```python
from build123d import *

# Parameters (mm, degrees)
F0_W          = 101.6
F0_H          = 76.2
F2_DEPTH      = 3.81
F3_DEPTH      = 38.1
F3_DEPTH_BACK = 38.1
F5_DEPTH      = 101.6
F6_R          = 2.032
F7_DEPTH      = 25.4
F9_R          = 3.175
F9_R_2        = 2.032
F10_DEPTH     = 25.4
F11_W         = 35.56
F11_H         = 25.4
F12_DEPTH     = 25.4
F13_T1_DEPTH  = 102.3282991577
F13_T3_DEPTH  = 70.6700590666
F13_T5_DEPTH  = 34.6541495789
F13_T11_DEPTH = 70.6700590666
F13_T16_DEPTH = 47.7182991577
F14_SIZE      = 5.08
F15_T1_DEPTH  = 71.0624204228
F15_T3_DEPTH  = 110.5507880402
F15_T5_DEPTH  = 71.0624204227
F16_R         = 5.08


# Not quite as in the source:
# - a fillet or chamfer that OpenCascade refuses, or shapes differently, is made with other operations: its cross-section is extruded or revolved along the edge and cut away or added


with BuildPart() as f2:
    # F0 (on Top) → F2 (new body)
    with BuildSketch(Plane.XY):
        with Locations((-38.1367237687, 0)):
            Rectangle(F0_W, F0_H)
    extrude(amount=F2_DEPTH)

    # F1 (on Front) → F3 (join, two sides)
    with BuildSketch(Plane.XZ) as f3_sk:
        Polygon((-44.9426332565, 25.4), (-88.9367237687, 0), (-44.9426332565, 0), align=None)
    extrude(amount=F3_DEPTH)
    extrude(f3_sk.sketch, amount=-F3_DEPTH_BACK)

    # F4 (on face) → F5 (cut)
    with BuildSketch(Plane.XZ.offset(38.1)):
        Polygon((-88.9367237687, 0), (-82.3376101919, 3.81), (-88.9367237687, 3.81), align=None)
    extrude(amount=-F5_DEPTH, mode=Mode.SUBTRACT)

    # F6 (on face) → F7 (cut)
    with BuildSketch(Plane(origin=(-22.2341809422, 0, 38.5107310565), x_dir=(0.8660254038, 0, 0.5), z_dir=(-0.5, 0, 0.8660254038))):
        with Locations((-69.4014621131, -13.4874)):
            Circle(F6_R)
        with Locations((-69.4014621131, -5.588)):
            Circle(F6_R)
        with Locations((-69.4014621131, 5.5626)):
            Circle(F6_R)
        with Locations((-69.4014621131, 13.462)):
            Circle(F6_R)
        with Locations((-42.4520621131, 13.462)):
            Circle(F6_R)
        with Locations((-42.4520621131, -5.588)):
            Circle(F6_R)
        with Locations((-42.4520621131, -13.4874)):
            Circle(F6_R)
        with Locations((-42.4520621131, 5.5626)):
            Circle(F6_R)
    extrude(amount=-F7_DEPTH, mode=Mode.SUBTRACT)

    # F9 (on offset) → F10 (cut)
    with BuildSketch(Plane(origin=(-20.3291809422, 0, 35.2111742681), x_dir=(0.8660254038, 0, 0.5), z_dir=(-0.5, 0, 0.8660254038))):
        with Locations((-69.4014621131, 13.462)):
            Circle(F9_R)
        with Locations((-69.4014621131, 13.462)):
            Circle(F9_R_2, mode=Mode.SUBTRACT)
        with Locations((-69.4014621131, 5.5626)):
            Circle(F9_R)
        with Locations((-69.4014621131, 5.5626)):
            Circle(F9_R_2, mode=Mode.SUBTRACT)
        with Locations((-69.4014621131, -5.588)):
            Circle(F9_R)
        with Locations((-69.4014621131, -5.588)):
            Circle(F9_R_2, mode=Mode.SUBTRACT)
        with Locations((-69.4014621131, -13.4874)):
            Circle(F9_R)
        with Locations((-69.4014621131, -13.4874)):
            Circle(F9_R_2, mode=Mode.SUBTRACT)
        with Locations((-42.4520621131, -5.588)):
            Circle(F9_R)
        with Locations((-42.4520621131, -5.588)):
            Circle(F9_R_2, mode=Mode.SUBTRACT)
        with Locations((-42.4520621131, -13.4874)):
            Circle(F9_R)
        with Locations((-42.4520621131, -13.4874)):
            Circle(F9_R_2, mode=Mode.SUBTRACT)
        with Locations((-42.4520621131, 5.5626)):
            Circle(F9_R)
        with Locations((-42.4520621131, 5.5626)):
            Circle(F9_R_2, mode=Mode.SUBTRACT)
        with Locations((-42.4520621131, 13.462)):
            Circle(F9_R)
        with Locations((-42.4520621131, 13.462)):
            Circle(F9_R_2, mode=Mode.SUBTRACT)
    extrude(amount=-F10_DEPTH, mode=Mode.SUBTRACT)

    # F11 (on face) → F12 (cut)
    with BuildSketch(Plane(origin=(0, 0, 0), x_dir=(1, 0, 0), z_dir=(0, 0, -1))):
        with Locations((-17.78, 0)):
            Rectangle(F11_W, F11_H)
    extrude(amount=-F12_DEPTH, mode=Mode.SUBTRACT)

    # F13: chamfer of 5.08 on 4 edges, made by hand

    # F13_s2 → F13_t1 (cut)
    with BuildSketch(Plane.XZ.offset(-51.1641495789)):
        Polygon((12.6632762313, -1.27), (7.5832762313, 3.81), (12.6632762313, 3.81), align=None)
    extrude(amount=F13_T1_DEPTH, mode=Mode.SUBTRACT)

    # F13_s4 → F13_t3 (cut)
    with BuildSketch(Plane.YZ.offset(-44.9426332565)):
        Polygon((-38.1, -1.27), (-33.02, 3.81), (-38.1, 3.81), align=None)
        Polygon((38.1, -1.27), (33.02, 3.81), (38.1, 3.81), align=None)
    extrude(amount=F13_T3_DEPTH, mode=Mode.SUBTRACT)

    # F13_s6 → F13_t5 (cut)
    with BuildSketch(Plane.XY.offset(3.81)):
        Polygon((-50.0226332565, 38.1), (-44.9426332565, 33.02), (-44.9426332565, 38.1), align=None)
    extrude(amount=F13_T5_DEPTH, mode=Mode.SUBTRACT)


with BuildPart() as f13_tool9:
    # F13_s10 → F13_t11 (new body)
    with BuildSketch(Plane.YZ.offset(12.6632762313)):
        Polygon((38.1, -1.27), (33.02, 3.81), (38.1, 3.81), align=None)
    extrude(amount=-F13_T11_DEPTH)

    split(bisect_by=Plane.XY, keep=Keep.TOP)

    split(bisect_by=Plane.YZ.offset(-44.9426332565), keep=Keep.BOTTOM)


with BuildPart() as f13_tool14:
    # F13_s15 → F13_t16 (new body)
    with BuildSketch(Plane.XY.offset(-9.2541495789)):
        Polygon((-50.0226332565, 38.1), (-44.9426332565, 33.02), (-44.9426332565, 38.1), align=None)
    extrude(amount=F13_T16_DEPTH)

    split(bisect_by=Plane.XY, keep=Keep.TOP)

    split(bisect_by=Plane.XY.offset(3.81), keep=Keep.BOTTOM)


with BuildPart() as f13_tool9_1:
    add(f13_tool9.part)

    # F13_t19: intersect F13_tool14
    add(f13_tool14.part, mode=Mode.INTERSECT)


with BuildPart() as f2_1:
    add(f2.part)

    # F13_t7: cut F13_tool9
    add(f13_tool9_1.part, mode=Mode.SUBTRACT)

    # F14
    f14_edges = [f2_1.edges().sort_by_distance(p)[0] for p in [
        (-44.942633, -38.1, 12.7),
    ]]
    chamfer(f14_edges, length=F14_SIZE)

    # F15: chamfer of 5.08 on 3 edges, made by hand

    # F15_s2 → F15_t1 (cut)
    with BuildSketch(Plane(origin=(-16.4745669001, 0, -9.5115956346), x_dir=(0, 1, 0), z_dir=(-0.8660254038, 0, -0.5))):
        Polygon((-38.1, -39.3883618844), (-33.02, -44.4683618844), (-38.1, -44.4683618844), align=None)
    extrude(amount=F15_T1_DEPTH, mode=Mode.SUBTRACT)

    # F15_s4 → F15_t3 (cut)
    with BuildSketch(Plane.XZ.offset(-55.2753940201)):
        Polygon((-52.5626332565, 21.0005909488), (-44.9426332565, 16.6011818976), (-44.9426332565, 25.4), align=None)
    extrude(amount=F15_T3_DEPTH, mode=Mode.SUBTRACT)

    # F15_s6 → F15_t5 (cut)
    with BuildSketch(Plane(origin=(-78.0164282407, 0, -45.042805846), x_dir=(0, 1, 0), z_dir=(0.8660254038, 0, 0.5))):
        Polygon((33.02, 44.4683618844), (38.1, 39.3883618844), (38.1, 44.4683618844), align=None)
    extrude(amount=F15_T5_DEPTH, mode=Mode.SUBTRACT)

    # F16
    f16_edges = [f2_1.edges().sort_by_distance(p)[0] for p in [
        (-35.56, -12.7, 1.905),
        (-35.56, 12.7, 1.905),
        (0, 12.7, 1.905),
        (0, -12.7, 1.905),
    ]]
    fillet(f16_edges, radius=F16_R)


solid = f2_1.part
```
Build history of the part. All positions in model axes, mm. A direction names the side the tool comes from. Give positions to 0.01 mm unless a question says otherwise; leave off trailing zeros. Loops run counter-clockwise (first coordinate to the right, second up) from the corner with the lowest first, then second, coordinate; pieces in that order, holes last. Notation, with made-up numbers: (21, 75.5) -> (57, 75.5) arc R30 ccw to (57, 106.5) -> close; hole circle Ø8 at (24, 86.5). An arc over 180 degrees is marked (long way). One line per question, with ' | ' between items. Start each with the question number.
1) Cut at A-A (x = -18). Give the cut face in (y, z).
2) Two-plate mould, pull along Y, no slides. Class faces 5 (the cylindrical face through (-34.111, 11.172, 1.932)), 6 (the flat face through (-58, 38.1, 5)), 7 (the flat face through (9.515, 0.516, 1.878)), 8 (the cylindrical face through (-50.04, 14.42, 7.82)): released by +Y, released by -Y, zero draft, split by the parting line, or undercut.
3) Cut at D-D (x = -3). Give the cut face in (y, z).
4) Probe L1, parallel to Y at x = -47.5, z = 2.25; L2, parallel to X at y = -8, z = 2; L3, parallel to Z at x = -36, y = 27.5. List the from-to ranges inside material, lowest first.
5) Cut at C-C (z = 6). Count the separate pieces of the cut face and the enclosed holes in it, plus the area to 3 significant figures.
6) 3-axis set-ups, long thin cutter, end or side, ignore diameter. For faces 1 (the flat face through (-39, 1, 0)), 2 (the flat face through (-19, 15, 3.81)), 3 (the flat face through (-18, -12.7, 2)), 4 (the flat face through (-55.3, 6.31, 15.02)): which of +Z, -Z, +X, -X, +Y, -Y reach the whole face in a straight line?
7) Cut at B-B (y = -21). Give the cut face in (x, z), plus the area to 3 significant figures.
8) Pin check, flat tips, straight feed: pin 1 (1.9 mm diameter, centred on x = -20, z = 1, fed in from +Y); pin 2 (5 mm diameter, centred on y = 28, z = 17.5, fed in from +X); pin 3 (5 mm diameter, centred on x = -74, y = -17.5, fed in from +Z). Stop position of each tip, or through.
Return value:
1) outline: (-36.83, 0) -> (-12.7, 0) -> (-12.7, 3.81) -> (-33.02, 3.81) -> close; (12.7, 0) -> (36.83, 0) -> (33.02, 3.81) -> (12.7, 3.81) -> close
2) face 5: undercut | face 6: released by +Y | face 7: zero draft | face 8: undercut
3) outline: (-36.83, 0) -> (-12.25, 0) -> (-12.25, 3.81) -> (-33.02, 3.81) -> close; (12.25, 0) -> (36.83, 0) -> (33.02, 3.81) -> (12.25, 3.81) -> close
4) L1: -35.58 to -15.52, -11.46 to -7.62, -3.56 to 3.53, 7.59 to 11.43, 15.49 to 35.58 | L2: -85.47 to -52.56, -47.79 to -35.55, -0.01 to 9.39 | L3: 0 to 3.81
5) separate pieces: 1 | enclosed holes: 4 | area: 2,340 mm^2
6) face 1: -Z, +X, -X, +Y, -Y | face 2: +Z, +X, +Y, -Y | face 3: +Z, -Z | face 4: none
7) outline: (-88.94, 0) -> (11.39, 0) -> (7.58, 3.81) -> (-44.94, 3.81) -> (-44.94, 16.6) -> (-52.56, 21) -> close | area: 733 mm^2
8) pin 1: y = 36.78 | pin 2: x = -44.94 | pin 3: z = 10.07
